Source: CAD feature listing. Evaluate the final solid. Frame: model axes, mm. A direction names the side the tool comes from. Coordinates: 2 decimals unless noted, no trailing zeros. Write each loop counter-clockwise with the first axis right and the second up, starting at its lowest first coordinate (ties: lowest second). Pieces come first, ordered by that corner, then holes. Notation, with made-up numbers: (-25, -8.5) - (31, -8.5) arc R15 ccw to (31, 9.5) - close; hole circle Ø9 at (29.5, 38). An arc over 180 degrees is marked (long way). One line per question, with ' | ' between items. Start each with the question number.
Q1. Cut plane C-C, the plane y = 13. Return loops of the section in (x, z), plus the area to 3 significant figures.
Q2. Cut plane B-B, the plane z = 18. Return loops of the section in (x, y).
Q3. Access query for faces 1 (the face through (-1, 50, 0)), 2 (the face through (28, 17, -6.576)). Directions: +Z, -Z, +X, -X, +Y, -Y. A direction counts if a zero-diameter tool reaches every point of the face in a straight line with its end or side. Return the directions, or none.
Q4. Line query: line 1 (Z direction, x = 18.5, y = 34.5); line 2 (Y direction, x = 7, z = 26.5); line 3 (X direction, y = 15.5, z = 6). Output: solid intervals per line, ascending.
Q5. Contact query for flat-ended pins moving along their axis: P1, Ø8, axis at x = 1, y = 21.5, coming from the +Z side; P2, Ø3, axis at y = 16, z = -1.5, coming from the +X side; P3, Ø1.5, axis at x = 21, z = 0, coming from the -Y side. Output: stop coordinate, or through.
Q6. Cut plane D-D, the plane x = -3.5. Return loops of the section in (y, z).
Q7. Cut plane A-A, the plane x = 46. Return loops of the section in (y, z).
```python
from build123d import *

# Parameters (mm, degrees)
F0_W     = 105
F0_H     = 65
F1_DEPTH = 50
F3_DEPTH = 40
F5_DEPTH = 25
F6_DEPTH = 25
F7_DEPTH = 25


# Not quite as in the source:
# - a feature names something its author has since deleted; it is built from what else it names


with BuildPart() as f1:
    # F0 (on Front) → F1 (new body)
    with BuildSketch(Plane.XZ):
        Rectangle(F0_W, F0_H)
    extrude(amount=-F1_DEPTH)

    # F2 (on face) → F3 (cut)
    with BuildSketch(Plane.YZ.offset(52.5)):
        Polygon((0, 32.5), (0, -6.5763359704), (35, -6.5763359704), (50, 32.5), align=None)
    extrude(amount=-F3_DEPTH, mode=Mode.SUBTRACT)

    # F4 (on face) → F5 (join)
    with BuildSketch(Plane.YZ.offset(12.5)):
        Polygon((34.35340128, 3.1539797953), (34.35340128, 32.5), (0, 32.5), (0, -6.5763359704), (17.5, -6.5763359704), align=None)
    extrude(amount=-F5_DEPTH)

    # F4 (on face) → F6 (join)
    with BuildSketch(Plane.YZ.offset(12.5)):
        Polygon((34.35340128, 3.1539797953), (34.35340128, 32.5), (0, 32.5), (0, -6.5763359704), (17.5, -6.5763359704), align=None)
    extrude(amount=-F6_DEPTH)

    # F4 (on face) → F7 (cut)
    with BuildSketch(Plane.YZ.offset(12.5)):
        Polygon((34.35340128, 3.1539797953), (34.35340128, 32.5), (0, 32.5), (0, -6.5763359704), (17.5, -6.5763359704), align=None)
    extrude(amount=-F7_DEPTH, mode=Mode.SUBTRACT)


solid = f1.part
```
Reply:
1) outline: (-52.5, -32.5) - (52.5, -32.5) - (52.5, -6.58) - (-12.5, -6.58) - (-12.5, 32.5) - (-52.5, 32.5) - close | area: 4,290 mm^2
2) outline: (-52.5, 0) - (-12.5, 0) - (-12.5, 34.35) - (12.5, 34.35) - (12.5, 44.43) - (52.5, 44.43) - (52.5, 50) - (-52.5, 50) - close
3) face 1: +Z, -Z, +X, -X, +Y | face 2: +Z, +X, -Y
4) line 1: z = -32.5 to -6.58 | line 2: y = 34.35 to 50 | line 3: x = -52.5 to -12.5
5) P1: stops at z = -1.96 | P2: stops at x = -12.5 | P3: stops at y = 37.24
6) outline: (0, -32.5) - (50, -32.5) - (50, 32.5) - (34.35, 32.5) - (34.35, 3.15) - (17.5, -6.58) - (0, -6.58) - close
7) outline: (0, -32.5) - (50, -32.5) - (50, 32.5) - (35, -6.58) - (0, -6.58) - close
